Autodesk Inventor part; units mm, degrees
ref_plane "YZ Plane" through (0, 0, 0) normal (1, 0, 0) x (0, 1, 0)
ref_plane "XZ Plane" through (0, 0, 0) normal (0, 1, 0) x (-1, 0, 0)
ref_plane "XY Plane" through (0, 0, 0) normal (0, 0, 1) x (1, 0, 0)
sketch "Sketch1" plane through (0, 0, 0) normal (1, 0, 0) x (0, 1, 0)
  arc A0 (25.215, 12.1739) -> (-25.215, 12.1739) centre (0, 0) ccw
  arc A1 (10.2581, 7.1429) -> (-10.2581, 7.1429) centre (0, 0) ccw
  circle A2 centre (0, 0) radius 1.5
  line L0 (-14.3614, 5) -> (-20.7123, 5)
  line L1 (14.3614, 5) -> (20.7123, 5)
  arc A3 (-25.215, 12.1739) -> (-20.7123, 5) centre (-20.7123, 10) ccw
  arc A4 (-14.3614, 5) -> (-10.2581, 7.1429) centre (-14.3614, 10) ccw
  arc A5 (10.2581, 7.1429) -> (14.3614, 5) centre (14.3614, 10) ccw
  arc A6 (20.7123, 5) -> (25.215, 12.1739) centre (20.7123, 10) ccw
  line L2 (27, -8.5) -> (-9, -8.5)
  line L3 (-12, -11.5) -> (-12, -8.988)
  arc A7 (-9, -8.5) -> (-12, -11.5) centre (-9, -11.5) ccw
  line L4 (-9, -19.5) -> (27, -19.5)
  line L5 (30, -16.5) -> (30, -11.5)
  circle A8 centre (0, 0) radius 46.5
  line L6 (-12, -11.5) -> (-12, -16.5)
  arc A9 (-12, -16.5) -> (-9, -19.5) centre (-9, -16.5) ccw
  arc A10 (27, -19.5) -> (30, -16.5) centre (27, -16.5) ccw
  arc A11 (30, -11.5) -> (27, -8.5) centre (27, -11.5) ccw
  point P0 (7.4416, -10.0435)
  point P1 (-11.4564, 5)
  point P2 (11.4564, 5)
  point P3 (-27.55, 5)
  point P4 (27.55, 5)
  dimension "d5" = 28
  dimension "d6" = 25
  dimension "d7" = 3
  dimension "d53" = 5
  dimension "d54" = 5
  dimension "d86" = 12
  dimension "d90" = 8.5
  dimension "d91" = 3
  dimension "d95" = 93
  dimension "d96" = 3
  dimension "d97" = 42
  dimension "d98" = 11
extrude "Extrusion3" add sketch "Sketch1" along normal blind 3
sketch "Sketch2" plane through (3, 0, 0) normal (1, 0, 0) x (0, 0, -1)
  arc A0 (-12.1739, 25.215) -> (-12.1739, -25.215) centre (0, 0) ccw
  line L0 (11, 43) -> (6, 43)
  line L1 (6, 43) -> (6, 40)
  line L2 (6, 40) -> (11, 40)
  line L3 (11, 40) -> (11, 43)
  dimension "d99" = 5
  dimension "d100" = 3
  dimension "d101" = 40
  dimension "d102" = 6
extrude "Extrusion5" cut sketch "Sketch2" against normal through all
sketch "Sketch4" plane through (3, 0, 0) normal (1, 0, 0) x (0, 0, -1)
  arc A0 (-12.1739, 25.215) -> (-12.1739, -25.215) centre (0, 0) ccw
  line L0 (-2, -20) -> (4, -20)
  line L1 (4, -20) -> (4, -25)
  line L2 (4, -25) -> (-2, -25)
  line L3 (-2, 22.5) -> (4, 22.5)
  line L4 (4, 22.5) -> (4, 12.5)
  line L5 (4, 12.5) -> (-2, 12.5)
  line L6 (-2, 22.5) -> (-2, 12.5)
  line L7 (-5, 20.7123) -> (-5, 14.3614)
  line L8 (-2, -20) -> (-2, -25)
  line L9 (6, 40) -> (6, 43)
  dimension "d59" = 5
  dimension "d60" = 20
  dimension "d62" = 10
  dimension "d63" = 12.5
  dimension "d94" = 6
  dimension "d104" = 2
extrude "Extrusion6" cut sketch "Sketch4" against normal through all
sketch "Sketch7" plane through (3, 0, 0) normal (1, 0, 0) x (0, 0, -1)
  line L0 (19.5, -6) -> (28, -6)
  line L1 (28, -6) -> (28, 6)
  line L2 (28, 6) -> (19.5, 6)
  line L3 (19.5, 6) -> (19.5, -6)
  line L4 (19.5, 27) -> (19.5, -9)
  point P0 (0, 0)
  point P1 (19.5, 0)
  dimension "d105" = 12
  dimension "d106" = 8.5
extrude "Extrusion9" cut sketch "Sketch7" against normal through all
fillet "Fillet1" radius 2 4 edges at (1.5, -6, -19.5) (1.5, -6, -28) (1.5, 6, -28) (1.5, 6, -19.5)
sketch "Sketch8" plane through (0, 0, 0) normal (-1, 0, 0) x (0, 0, 1)
  line L0 (-37, 7) -> (-29, 7)
  line L1 (-29, 7) -> (-29, 19)
  line L2 (-29, 19) -> (-37, 19)
  line L3 (-37, 19) -> (-37, 7)
  point P0 (0, 0)
  dimension "d110" = 12
  dimension "d111" = 8
  dimension "d112" = 29
  dimension "d113" = 7
extrude "Extrusion10" cut sketch "Sketch8" against normal through all
fillet "Fillet2" radius 1 4 edges at (1.5, 7, -29) (1.5, 7, -37) (1.5, 19, -37) (1.5, 19, -29)
sketch "Sketch9" plane through (0, 0, 0) normal (-1, 0, 0) x (0, 0, 1)
  circle A0 centre (-22.5, -21) radius 5
  point P0 (0, 0)
  dimension "d117" = 10
  dimension "d118" = 22.5
  dimension "d119" = 21
extrude "Extrusion11" cut sketch "Sketch9" against normal through all
properties part number "2.8chassis side DB25V3"
Verification items for the finished model (mm, model axes). Coordinates: 2 decimals unless noted, no trailing zeros. Write each loop counter-clockwise with the first axis right and the second up, starting at its lowest first coordinate (ties: lowest second). Pieces come first, ordered by that corner, then holes. Notation, with made-up numbers: M 20.25,50.5 L 24.25,50.5 A20 cw 24.25,80.5 Z; hole C -17,2.25 d6. An arc over 180 degrees is marked long. Use CSV: the item, a comma, the result in double quotes.
Q1. Thickness scan on line 1 along Z through (x, y) = (2.65, -11); line 2 along Z through (x, y) = (1.25, 4.5); line 3 along Y through (x, z) = (2.6, -24.5). Record the ranges inside material, lowest first. Write a range as [from, to].
Computed values:
line 1,"[-45.18, -18.74], [-9.26, 6.3], [25.75, 45.18]"
line 2,"[-46.28, -27.94], [-8.5, 11.66], [27.64, 46.28]"
line 3,"[-39.52, -25.58], [-16.42, -6], [6, 39.52]"
Q2. Section check C-C, the plane x = 1.4. State how many separate pieces and enclosed holes the cut face has, and give its area (3 significant figures).
Computed values:
separate pieces,"1"
enclosed holes,"8"
area,"5,150 mm²"
Q3. Go/stop test with flat-tipped pins: P1, Ø1.5, axis at x = 1.5, z = -2, coming from the -Y side; P2, Ø1.8, axis at y = 0, z = 0, coming from the -X side; P3, Ø0.9, axis at x = 1, z = -24.5, coming from the -Y side; P4, Ø1.5, axis at x = 2, y = 20.5, coming from the +Z side. Record where each tip stops, or that it passes through.
Computed values:
P1,"y = -46.48"
P2,"through"
P3,"y = -39.8"
P4,"z = 42.1"
Q4. Section check D-D, the plane y = -33. Enter the section's corners in (x, z), and give its area (3 significant figures).
Computed values:
outline,"M 0,-32.76 L 3,-32.76 L 3,32.76 L 0,32.76 Z"
area,"197 mm²"
Q5. Section check A-A, the plane y = 0. Enter the section's corners in (x, z), and give its area (3 significant figures).
Computed values:
outline,"M 0,-46.5 L 3,-46.5 L 3,-28 L 0,-28 Z; M 0,-8.5 L 3,-8.5 L 3,-1.5 L 0,-1.5 Z; M 0,1.5 L 3,1.5 L 3,12.5 L 0,12.5 Z; M 0,28 L 3,28 L 3,46.5 L 0,46.5 Z"
area,"165 mm²"
Q6. Section check B-B, the plane z = 18. Enter the section's corners in (x, y), and give its area (3 significant figures).
Computed values:
outline,"M 0,-42.87 L 3,-42.87 L 3,-21.45 L 0,-21.45 Z; M 0,21.45 L 3,21.45 L 3,42.87 L 0,42.87 Z"
area,"129 mm²"
Q7. Mould release check, pull along Z, two halves, no side actions. Record for faces 1 (the flat face through (3, 10, 1)), 2 (the cylindrical face through (1.48, 44.35, -13.97)), 3 (the cylindrical face through (1.48, 5.43, -27.4)): pulls with the +Z half, pulls with the -Z half, needs draft (parallel to the pull), parting line crosses it, or undercut.
Computed values:
face 1,"needs draft"
face 2,"parting line crosses it"
face 3,"undercut"
